For this review, use the dimensioned drawing (mm, ordinates from the lowest corner) and the shaded views. A direction names the side the tool comes from. Coordinates: 2 decimals unless noted, no trailing zeros. Order: outer loops, then holes, each group sorted by start corner. A loop starts at its lowest first (then second) coordinate and runs counter-clockwise, first axis right, second up. Notation, with made-up numbers: M 21.25,37.5 L 75.25,37.5 A28 cw 75.25,61.5 Z; hole C 54,-13 d6. An arc over 180 degrees is marked long. Answer in a Markdown table with one row per item.
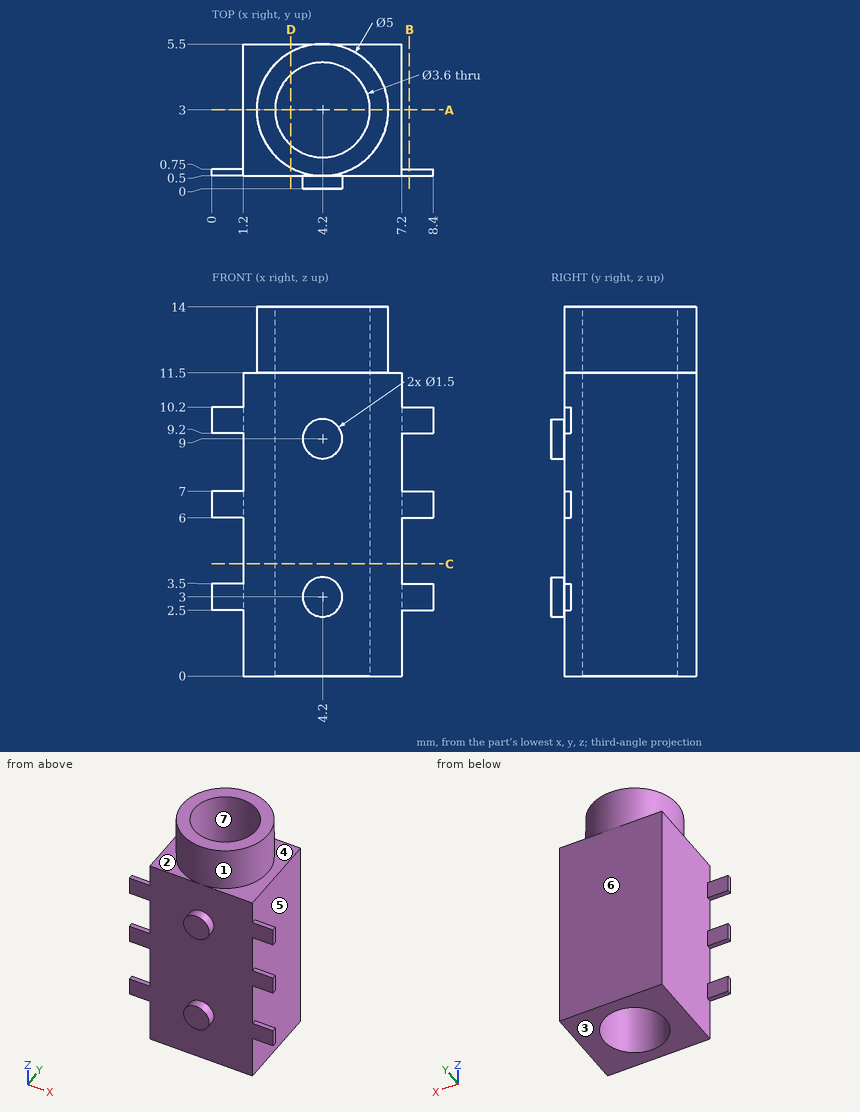
(1) Insertion check: pin 1 Ø1.5 at (x, y) = (1, 2) entering from +Z; pin 2 Ø0.8 at (x, z) = (0.5, 6.5) entering from +Y. Each pin has a flat end and moves straight along its axis. Give the tip position at first contact, or say it passes through.
Return value:
| item | result |
|---|---|
| pin 1 | stops at z = 11.5 |
| pin 2 | stops at y = 0.75 |
(2) Add section C-C, the plane z = 4.25. Give the boundary of the cut face in (x, y).
Return value:
| item | result |
|---|---|
| outline | M 1.2,0.5 L 7.2,0.5 L 7.2,5.5 L 1.2,5.5 Z; hole C 4.2,3 d3.6 |
(3) Add section B-B, the plane x = 7.5. Give the boundary of the cut face in (y, z), and give its area (3 significant figures).
Return value:
| item | result |
|---|---|
| outline | M 0.5,2.5 L 0.75,2.5 L 0.75,3.5 L 0.5,3.5 Z; M 0.5,6 L 0.75,6 L 0.75,7 L 0.5,7 Z; M 0.5,9.2 L 0.75,9.2 L 0.75,10.2 L 0.5,10.2 Z |
| area | 0.750 mm2 |
(4) Add section D-D, the plane x = 3. Give the boundary of the cut face in (y, z).
Return value:
| item | result |
|---|---|
| outline | M 0.5,0 L 1.66,0 L 1.66,14 L 0.81,14 L 0.81,11.5 L 0.5,11.5 Z; M 4.34,0 L 5.5,0 L 5.5,11.5 L 5.19,11.5 L 5.19,14 L 4.34,14 Z |
(5) For line 1 along Y through (x, z) = (4.2, 7.75); line 2 along X through (y, z) = (3.05, 10.5); line 3 along Y through (x, z) = (4.2, 3.25), list the stretches that pass through material, from the lowest coordinate up. Write a range as from..to.
Return value:
| item | result |
|---|---|
| line 1 | y = 0.5..1.2, 4.8..5.5 |
| line 2 | x = 1.2..2.4, 6..7.2 |
| line 3 | y = 0..1.2, 4.8..5.5 |
(6) Draft analysis for pull direction Y (two halves, no side actions). For the marked faces 5, 6 and 7, state which applies: pulls with the +Y half, pulls with the -Y half, needs draft (parallel to the pull), parting line crosses it, or undercut.
Return value:
| item | result |
|---|---|
| face 5 | needs draft |
| face 6 | pulls with the +Y half |
| face 7 | undercut |
(7) Add section A-A, the plane y = 3. Give the boundary of the cut face in (x, z).
Return value:
| item | result |
|---|---|
| outline | M 1.2,0 L 2.4,0 L 2.4,14 L 1.7,14 L 1.7,11.5 L 1.2,11.5 Z; M 6,0 L 7.2,0 L 7.2,11.5 L 6.7,11.5 L 6.7,14 L 6,14 Z |
(8) For the marked faces 1, 2, 3 and 4, list the 3-axis set-ups (+Z, -Z, +X, -X, +Y, -Y) from which the entire face can be reached by the end or side of a thin tool; tool diameter is ignored.
Return value:
| item | result |
|---|---|
| face 1 | +Z |
| face 2 | +Z, -X |
| face 3 | -Z, +X, -X, +Y, -Y |
| face 4 | +Z, +X |
